Source: CAD feature listing. Evaluate the final solid. Frame: model axes, mm. Round coordinates to 2 decimals unless told otherwise and drop trailing zeros. Write each loop counter-clockwise with the first axis right and the second up, starting at its lowest first coordinate (ties: lowest second). Pieces come first, ordered by that corner, then holes. Notation, with made-up numbers: M 68,62 L 79,62 A18 cw 79,73 Z; hole C 72.5,36 d9. An arc over 180 degrees is marked long. Use a Markdown table: item, result.
```python
from build123d import *

# Parameters (mm, degrees)
BODYSKE_R   = 0.6
BODY_DEPTH  = 0.8
NOTSKE_W    = 2
NOTSKE_H    = 1.2
NOTCH_DEPTH = 1.8


with BuildPart() as part:
    # BodySke → Body (new body)
    with BuildSketch(Plane.XY):
        with BuildLine():
            Line((0.108571429, -3.798448663), (0.2, -6.997142274))
            ThreePointArc((0.2, -6.997142274), (0.887407187, -6.943522772), (1.566204647, -6.822536405))
            ThreePointArc((1.566204647, -6.822536405), (1.953248067, -6.596169328), (2.141980652, -6.189445006))
            Line((2.141980652, -6.189445006), (2.321707775, -4.824281977))
            ThreePointArc((2.321707775, -4.824281977), (2.597941642, -3.974889916), (3.160591953, -3.281206522))
            ThreePointArc((3.160591953, -3.281206522), (0, 5.3), (-3.160591953, -3.281206522))
            ThreePointArc((-3.160591953, -3.281206522), (-2.597941642, -3.974889916), (-2.321707775, -4.824281977))
            Line((-2.321707775, -4.824281977), (-2.141980652, -6.189445006))
            ThreePointArc((-2.141980652, -6.189445006), (-1.953248067, -6.596169328), (-1.566204647, -6.822536405))
            ThreePointArc((-1.566204647, -6.822536405), (-0.887407187, -6.943522772), (-0.2, -6.997142274))
            Line((-0.2, -6.997142274), (-0.108571429, -3.798448663))
            ThreePointArc((-0.108571429, -3.798448663), (0, 3.8), (0.108571429, -3.798448663))
        make_face()
        with Locations((1, -5.408326913)):
            Circle(BODYSKE_R, mode=Mode.SUBTRACT)
        with Locations((-1, -5.408326913)):
            Circle(BODYSKE_R, mode=Mode.SUBTRACT)
    extrude(amount=-BODY_DEPTH)

    # NotSke → Notch (cut, through all)
    with BuildSketch(Plane.XY):
        with Locations((0, -5.408326913)):
            Rectangle(NOTSKE_W, NOTSKE_H)
    extrude(amount=-NOTCH_DEPTH, mode=Mode.SUBTRACT)


solid = part.part
```
Q1. Section A-A on z = -0.55. Return loops of the section in (x, y).
Results are:
| item | result |
|---|---|
| outline | M -3.16,-3.28 A2.45 cw -2.32,-4.82 L -2.14,-6.19 A0.75 ccw -1.57,-6.82 A7 ccw -0.2,-7 L -0.17,-6.01 L -1,-6.01 A0.6 cw -1,-4.81 L -0.14,-4.81 L -0.11,-3.8 A3.8 cw long 0.11,-3.8 L 0.14,-4.81 L 1,-4.81 A0.6 cw 1,-6.01 L 0.17,-6.01 L 0.2,-7 A7 ccw 1.57,-6.82 A0.75 ccw 2.14,-6.19 L 2.32,-4.82 A2.45 cw 3.16,-3.28 A4.87 ccw long Z |
Q2. Line query: L1, parallel to Y at x = 1.25, z = -0.7; L2, parallel to Y at x = -0.5, z = -0.3; L3, parallel to X at y = 0, z = -0.25. Output: solid intervals per line, ascending.
Results are:
| item | result |
|---|---|
| L1 | -6.89 to -5.95, -4.86 to -3.59, 3.59 to 5.14 |
| L2 | -6.98 to -6.01, -4.81 to -3.77, 3.77 to 5.27 |
| L3 | -4.85 to -3.8, 3.8 to 4.85 |
Q3. Mould query, pull axis Y, two halves, no side actions, for faces 1 (the cylindrical face through (-0.166, 3.796, -0.394)), 2 (the cylindrical face through (0.166, 5.297, -0.394)), 3 (the cylindrical face through (2.59, -3.99, -0.39)). Classes: +Y half, -Y half, draft (parallel to the pull), parting line (faces both ways), or undercut.
Results are:
| item | result |
|---|---|
| face 1 | undercut |
| face 2 | parting line |
| face 3 | -Y half |
Q4. Section B-B on y = -2.75. Return loops of the section in (x, z), plus the area to 3 significant figures.
Results are:
| item | result |
|---|---|
| outline | M -3.69,-0.8 L -2.62,-0.8 L -2.62,0 L -3.69,0 Z; M 2.62,-0.8 L 3.69,-0.8 L 3.69,0 L 2.62,0 Z |
| area | 1.71 mm^2 |
Q5. Section C-C on x = -3. Return loops of the section in (y, z).
Results are:
| item | result |
|---|---|
| outline | M -3.43,-0.8 L -2.33,-0.8 L -2.33,0 L -3.43,0 Z; M 2.33,-0.8 L 4.27,-0.8 L 4.27,0 L 2.33,0 Z |
